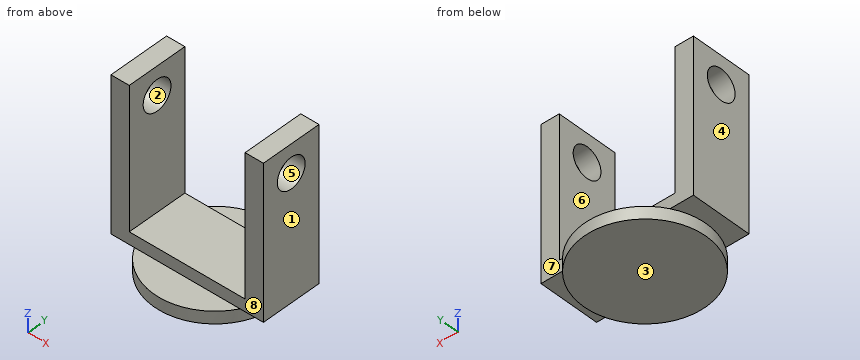
```python
from build123d import *

# Parameters (mm, degrees)
SKETCH1_R           = 50
BOSS_EXTRUDE1_DEPTH = 10
SKETCH2_W           = 125
SKETCH2_H           = 50
BOSS_EXTRUDE2_DEPTH = 10
SKETCH3_W           = 15
SKETCH3_H           = 50
BOSS_EXTRUDE3_DEPTH = 115
SKETCH4_R           = 12.5
CUT_EXTRUDE1_DEPTH  = 126


with BuildPart() as part:
    # Sketch1 → Boss-Extrude1 (new body)
    with BuildSketch(Plane.XY):
        Circle(SKETCH1_R)
    extrude(amount=BOSS_EXTRUDE1_DEPTH)

    # Sketch2 → Boss-Extrude2 (add)
    with BuildSketch(Plane.XY.offset(10)):
        Rectangle(SKETCH2_W, SKETCH2_H)
    extrude(amount=BOSS_EXTRUDE2_DEPTH)

    # Sketch3 → Boss-Extrude3 (add)
    with BuildSketch(Plane.XY.offset(20)):
        with Locations((-55, 0)):
            Rectangle(SKETCH3_W, SKETCH3_H)
        with Locations((55, 0)):
            Rectangle(SKETCH3_W, SKETCH3_H)
    extrude(amount=BOSS_EXTRUDE3_DEPTH)

    # Sketch4 → Cut-Extrude1 (cut, through all)
    with BuildSketch(Plane.ZY.offset(62.5)):
        with Locations((112, 0)):
            Circle(SKETCH4_R)
    extrude(amount=-CUT_EXTRUDE1_DEPTH, mode=Mode.SUBTRACT)


solid = part.part
```
Can you work these out from the model? Positions are in its coordinate system, mm. Face numbers are marked on the shaded views. A direction names the side the tool comes from. Give positions to 0.01 mm unless a question says otherwise; leave off trailing zeros. Loops run counter-clockwise (first coordinate to the right, second up) from the corner with the lowest first, then second, coordinate; pieces in that order, holes last. Notation, with made-up numbers: M 64,49.5 L 86,49.5 A26 ccw 86,66.5 Z; hole C 57.25,4.25 d3. An arc over 180 degrees is marked long. Answer in a Markdown table with one row per item.
1. If I drill on line 1 along Y through (x, z) = (-50.75, 112); line 2 along X through (y, z) = (10, 125); line 3 along Z through (x, y) = (16, -15), over which ranges is the centre line in solid material (lowest first)?
Taken from the geometry:
| item | result |
|---|---|
| line 1 | y = -25 to -12.5, 12.5 to 25 |
| line 2 | x = -62.5 to -47.5, 47.5 to 62.5 |
| line 3 | z = 0 to 20 |
2. Suppose I cut it at A-A on z = 112. Write out the boundary of the cut face in (x, y), plus the area to 3 significant figures.
Taken from the geometry:
| item | result |
|---|---|
| outline | M -62.5,-25 L -47.5,-25 L -47.5,-12.5 L -62.5,-12.5 Z; M -62.5,12.5 L -47.5,12.5 L -47.5,25 L -62.5,25 Z; M 47.5,-25 L 62.5,-25 L 62.5,-12.5 L 47.5,-12.5 Z; M 47.5,12.5 L 62.5,12.5 L 62.5,25 L 47.5,25 Z |
| area | 750 mm² |
3. For pin 1 Ø12.5 at (x, y) = (5, -43.5) entering from +Z; pin 2 Ø22.5 at (y, z) = (0, 112) entering from -X; pin 3 Ø25 at (y, z) = (1.5, 100) entering from +X; pin 4 Ø12 at (x, z) = (50, 96) entering from +Y, each with a flat end and sliding along its axis, tell me the tip position at first contact or that it passes through.
Taken from the geometry:
| item | result |
|---|---|
| pin 1 | stops at z = 10 |
| pin 2 | passes through |
| pin 3 | stops at x = 62.5 |
| pin 4 | stops at y = 25 |
4. Thinking about a two-plate mould opening in Z: for the marked faces 1, 2 and 3, which applies, released by +Z, released by -Z, zero draft, split by the parting line, or undercut?
Taken from the geometry:
| item | result |
|---|---|
| face 1 | zero draft |
| face 2 | undercut |
| face 3 | released by -Z |
5. Suppose I cut it at D-D on x = 40. Write out the boundary of the cut face in (y, z), plus the area to 3 significant figures.
Taken from the geometry:
| item | result |
|---|---|
| outline | M -30,0 L 30,0 L 30,10 L 25,10 L 25,20 L -25,20 L -25,10 L -30,10 Z |
| area | 1,100 mm² |
6. Which directions (+Z, -Z, +X, -X, +Y, -Y) give clear straight access to the entire face, cutting with the end or side of a thin tool? Please do the marked faces 4, 5, 6, 7 and 8.
Taken from the geometry:
| item | result |
|---|---|
| face 4 | +Z, -Z, -X, +Y, -Y |
| face 5 | +X, -X |
| face 6 | +Z, +Y, -Y |
| face 7 | +Z, +X, -X, +Y |
| face 8 | +Z, +X, -X, -Y |
7. Suppose I cut it at C-C on z = 97. Write out the boundary of the cut face in (x, y).
Taken from the geometry:
| item | result |
|---|---|
| outline | M -62.5,-25 L -47.5,-25 L -47.5,25 L -62.5,25 Z; M 47.5,-25 L 62.5,-25 L 62.5,25 L 47.5,25 Z |
8. Suppose I cut it at B-B on y = 0. Write out the boundary of the cut face in (x, z).
Taken from the geometry:
| item | result |
|---|---|
| outline | M -62.5,10 L -50,10 L -50,0 L 50,0 L 50,10 L 62.5,10 L 62.5,99.5 L 47.5,99.5 L 47.5,20 L -47.5,20 L -47.5,99.5 L -62.5,99.5 Z; M -62.5,124.5 L -47.5,124.5 L -47.5,135 L -62.5,135 Z; M 47.5,124.5 L 62.5,124.5 L 62.5,135 L 47.5,135 Z |
